Read the model definition and answer for the solid it produces. Units are mm, in the model's axes. A direction names the side the tool comes from. Give positions to 0.01 mm unless a question says otherwise; leave off trailing zeros. Loops run counter-clockwise (first coordinate to the right, second up) from the corner with the lowest first, then second, coordinate; pieces in that order, holes last. Notation, with made-up numbers: (3.5, 14) - (42.5, 14) arc R17 ccw to (42.5, 20) - close; hole circle Ø7 at (-37, 10.25). An arc over 180 degrees is marked (long way). Use a Markdown table: item, result. Add a question column.
Item 1: A cutting plane is placed at A-A (y = 124.5). Determine the outline of the cut face in (x, z).
Item 2: Which of the six approach directions +Z, -Z, +X, -X, +Y, -Y give full straight-line access (tool end or side, diameter ignored) to faces 1 (the face through (128.614, 56.311, 3.944)), 2 (the face through (37.56, 139.12, 4.54)), 3 (the face through (70, 0, 4))?
Item 3: For a pull along Z with two mould halves and no side action, classify faces 4 (the face through (71, 73, 8)), 5 (the face through (137, 134.052, 4)), 6 (the face through (140.936, 27.363, 3.944)) as +Z half, -Z half, draft (parallel to the pull), parting line (faces both ways), or undercut.
Item 4: A cutting plane is placed at B-B (x = 70). Determine the outline of the cut face in (y, z).
Item 5: A cutting plane is placed at C-C (y = 56.5). Determine the outline of the cut face in (x, z), plus the area to 3 significant figures.
Item 6: Consider probe 1 along X at (y, z) = (78, 0.75); probe 2 along Y at (x, z) = (117, 2); probe 3 along Y at (x, z) = (100.5, 1.75). Determine where each line is inside the solid, lowest interval first. Write a range as [from, to].
Item 7: A cutting plane is placed at D-D (x = 40). Determine the outline of the cut face in (y, z).
Item 8: Each of these flat-tipped pins is pushed along its axis until it touches: P1, Ø2, axis at x = 46.5, z = 2, coming from the -Y side; P2, Ø1.5, axis at x = 101, z = 3.5, coming from the +Y side; P3, Ø0.9, axis at x = 123.5, z = 5.5, coming from the +Y side. Where does it stop, or does it pass through?
from build123d import *

# Parameters (mm, degrees)
BOSS_EXTRUDE1_DEPTH    = 8
SPLIT1_SURFACE_1_BACK  = 343.199
SPLIT1_SURFACE_1_DEPTH = 686.398
SPLIT1_SURFACE_2_BACK  = 343.199
SPLIT1_SURFACE_2_DEPTH = 686.398
SKETCH5_R              = 2.5
CUT_EXTRUDE6_DEPTH     = 10
SKETCH4_R              = 2.5
CUT_EXTRUDE7_DEPTH     = 10
SKETCH6_R              = 1.5
CUT_EXTRUDE8_DEPTH     = 342.206659287
SKETCH7_W              = 49
SKETCH7_H              = 49
SKETCH7_W_2            = 18
SKETCH7_H_2            = 18
BOSS_EXTRUDE2_DEPTH    = 15
SKETCH8_W              = 49
SKETCH8_H              = 49
SKETCH8_R              = 1.5
BOSS_EXTRUDE3_DEPTH    = 10
SKETCH9_W              = 49
SKETCH9_H              = 49
CUT_EXTRUDE9_DEPTH     = 8
SKETCH10_W             = 49
SKETCH10_H             = 49
SKETCH10_W_2           = 18
SKETCH10_H_2           = 18
BOSS_EXTRUDE4_DEPTH    = 8
SKETCH12_R             = 2.5
CUT_EXTRUDE10_DEPTH    = 343.027753759


with BuildPart() as part:
    # Sketch1 → Boss-Extrude1 (new body)
    with BuildSketch(Plane.XY):
        with BuildLine():
            Line((70, 309.985818768), (85.299227191, 309.985818768))
            ThreePointArc((85.299227191, 309.985818768), (88.489017574, 308.836174247), (90.211957942, 305.915913694))
            Line((90.211957942, 305.915913694), (96.672728921, 271.790334282))
            ThreePointArc((96.672728921, 271.790334282), (97.06575438, 270.906904614), (97.621470019, 270.115641625))
            Line((97.621470019, 270.115641625), (139.950460317, 220.786053348))
            ThreePointArc((139.950460317, 220.786053348), (141.739336996, 217.746026552), (142.361429131, 214.274017901))
            Line((142.361429131, 214.274017901), (142.361429131, 30.859943174))
            ThreePointArc((142.361429131, 30.859943174), (140.896963037, 27.324409268), (137.361429131, 25.859943174))
            Line((137.361429131, 25.859943174), (114.717190871, 25.782318449))
            ThreePointArc((114.717190871, 25.782318449), (112.681998989, 25.341726514), (111.002773989, 24.110332733))
            Line((111.002773989, 24.110332733), (89.38285929, 0))
            Line((89.38285929, 0), (50.5, 0))
            Line((50.5, 0), (28.997226011, 24.110332733))
            ThreePointArc((28.997226011, 24.110332733), (27.318001011, 25.341726514), (25.282809129, 25.782318449))
            Line((25.282809129, 25.782318449), (2.638570869, 25.859943174))
            ThreePointArc((2.638570869, 25.859943174), (-0.896963037, 27.324409268), (-2.361429131, 30.859943174))
            Line((-2.361429131, 30.859943174), (-2.361429131, 214.274017901))
            ThreePointArc((-2.361429131, 214.274017901), (-1.739336996, 217.746026552), (0.049539683, 220.786053348))
            Line((0.049539683, 220.786053348), (42.261389271, 270.115641625))
            ThreePointArc((42.261389271, 270.115641625), (42.81710491, 270.906904614), (43.210130369, 271.790334282))
            Line((43.210130369, 271.790334282), (49.724618218, 305.923183314))
            ThreePointArc((49.724618218, 305.923183314), (51.449026762, 308.838533573), (54.635967087, 309.985818768))
            Line((54.635967087, 309.985818768), (70, 309.985818768))
        make_face()
        with BuildLine():
            Line((15.218798766, 54.807228462), (17.702103505, 54.807228462))
            ThreePointArc((17.702103505, 54.807228462), (21.420312934, 56.347361236), (22.960445707, 60.065570665))
            Line((22.960445707, 60.065570665), (22.960445707, 189.807228462))
            ThreePointArc((22.960445707, 189.807228462), (21.495979613, 193.342762368), (17.960445707, 194.807228462))
            Line((17.960445707, 194.807228462), (14.960456564, 194.807228462))
            ThreePointArc((14.960456564, 194.807228462), (11.424922658, 193.342762368), (9.960456564, 189.807228462))
            Line((9.960456564, 189.807228462), (9.960456564, 60.065570665))
            ThreePointArc((9.960456564, 60.065570665), (11.500589337, 56.347361236), (15.218798766, 54.807228462))
        make_face(mode=Mode.SUBTRACT)
        with BuildLine():
            Line((125.039543436, 54.807228462), (122.039554293, 54.807228462))
            ThreePointArc((122.039554293, 54.807228462), (118.504020387, 56.271694556), (117.039554293, 59.807228462))
            Line((117.039554293, 59.807228462), (117.039554293, 189.807228462))
            ThreePointArc((117.039554293, 189.807228462), (118.504020387, 193.342762368), (122.039554293, 194.807228462))
            Line((122.039554293, 194.807228462), (125.039543436, 194.807228462))
            ThreePointArc((125.039543436, 194.807228462), (128.575077342, 193.342762368), (130.039543436, 189.807228462))
            Line((130.039543436, 189.807228462), (130.039543436, 59.807228462))
            ThreePointArc((130.039543436, 59.807228462), (128.575077342, 56.271694556), (125.039543436, 54.807228462))
        make_face(mode=Mode.SUBTRACT)
    extrude(amount=BOSS_EXTRUDE1_DEPTH)


with BuildPart() as body_2:
    # Split1: the piece behind the surface
    add(part.part)
    # Split1 surface: a surface, the sketch's curves swept straight by 686.398 mm
    with BuildLine(Plane(origin=(0, 0, 0), x_dir=(-1, 0, 0), z_dir=(0, 0, -1)).offset(-SPLIT1_SURFACE_1_BACK), mode=Mode.PRIVATE) as split1_surface_1_path:
        Line((-142.361429131, 144.05225917), (2.361429131, 144.05225917))
    split1_surface_1 = Shell.extrude(split1_surface_1_path.wire(), (0 * SPLIT1_SURFACE_1_DEPTH, 0 * SPLIT1_SURFACE_1_DEPTH, -1 * SPLIT1_SURFACE_1_DEPTH))
    split(bisect_by=split1_surface_1, keep=Keep.BOTTOM)

    # Sketch5 → Cut-Extrude6 (cut)
    with BuildSketch(Plane(origin=(0, 144.05225917, -115.359943174), x_dir=(1, 0, 0), z_dir=(0, -1, 0))):
        with Locations(Location((70, 119.359943174, 0), (0, 0, 270))):
            Circle(SKETCH5_R)
        with Locations(Location((100, 119.359943174, 0), (0, 0, 270))):
            Circle(SKETCH5_R)
        with Locations(Location((40, 119.359943174, 0), (0, 0, 270))):
            Circle(SKETCH5_R)
        with Locations(Location((2.638570869, 119.359943174, 0), (0, 0, 270))):
            Circle(SKETCH5_R)
        with Locations(Location((137.361429131, 119.359943174, 0), (0, 0, 270))):
            Circle(SKETCH5_R)
    extrude(amount=CUT_EXTRUDE6_DEPTH, mode=Mode.SUBTRACT)


with BuildPart() as part_1:
    add(part.part)

    # Split1: split by a surface, the side it looks to stays
    # Split1 surface: a surface, the sketch's curves swept straight by 686.398 mm
    with BuildLine(Plane(origin=(0, 0, 0), x_dir=(-1, 0, 0), z_dir=(0, 0, -1)).offset(-SPLIT1_SURFACE_2_BACK), mode=Mode.PRIVATE) as split1_surface_2_path:
        Line((-142.361429131, 144.05225917), (2.361429131, 144.05225917))
    split1_surface_2 = Shell.extrude(split1_surface_2_path.wire(), (0 * SPLIT1_SURFACE_2_DEPTH, 0 * SPLIT1_SURFACE_2_DEPTH, -1 * SPLIT1_SURFACE_2_DEPTH))
    split(bisect_by=split1_surface_2, keep=Keep.TOP)

    # Sketch4 → Cut-Extrude7 (cut)
    with BuildSketch(Plane(origin=(0, 144.05225917, 0), x_dir=(-1, 0, 0), z_dir=(0, -1, 0))):
        with Locations(Location((-70, -4, 0), (0, 0, 90))):
            Circle(SKETCH4_R)
        with Locations(Location((-40, -4, 0), (0, 0, 90))):
            Circle(SKETCH4_R)
        with Locations(Location((-100, -4, 0), (0, 0, 90))):
            Circle(SKETCH4_R)
        with Locations(Location((-137.361429131, -4, 0), (0, 0, 90))):
            Circle(SKETCH4_R)
        with Locations(Location((-3.799513716, -4, 0), (0, 0, 270))):
            Circle(SKETCH4_R)
    extrude(amount=-CUT_EXTRUDE7_DEPTH, mode=Mode.SUBTRACT)

    # Sketch6 → Cut-Extrude8 (cut, through all)
    with BuildSketch(Plane.XY.offset(8)):
        with Locations((50.000130369, 267.980334282)):
            Circle(SKETCH6_R)
        with Locations((90.000130369, 267.980334282)):
            Circle(SKETCH6_R)
        with Locations((90.000130369, 227.980334282)):
            Circle(SKETCH6_R)
        with Locations((50.000130369, 227.980334282)):
            Circle(SKETCH6_R)
    extrude(amount=-CUT_EXTRUDE8_DEPTH, mode=Mode.SUBTRACT)

    # Sketch7 → Boss-Extrude2 (add)
    with BuildSketch(Plane(origin=(0, 0, 0), x_dir=(-1, 0, 0), z_dir=(0, 0, -1))):
        with Locations((-70.000130369, 247.980334282)):
            Rectangle(SKETCH7_W, SKETCH7_H)
        with Locations((-56.000130369, 261.980334282)):
            Rectangle(SKETCH7_W_2, SKETCH7_H_2, mode=Mode.SUBTRACT)
        with Locations((-84.000130369, 261.980334282)):
            Rectangle(SKETCH7_W_2, SKETCH7_H_2, mode=Mode.SUBTRACT)
        with Locations((-84.000130369, 233.980334282)):
            Rectangle(SKETCH7_W_2, SKETCH7_H_2, mode=Mode.SUBTRACT)
        with Locations((-56.000130369, 233.980334282)):
            Rectangle(SKETCH7_W_2, SKETCH7_H_2, mode=Mode.SUBTRACT)
    extrude(amount=BOSS_EXTRUDE2_DEPTH)

    # Sketch8 → Boss-Extrude3 (add)
    with BuildSketch(Plane(origin=(0, 0, -15), x_dir=(-1, 0, 0), z_dir=(0, 0, -1))):
        with Locations((-70.000130369, 247.980334282)):
            Rectangle(SKETCH8_W, SKETCH8_H)
        with Locations(Location((-50.000130369, 267.980334282, 0), (0, 0, 180))):
            Circle(SKETCH8_R, mode=Mode.SUBTRACT)
        with Locations(Location((-90.000130369, 267.980334282, 0), (0, 0, 180))):
            Circle(SKETCH8_R, mode=Mode.SUBTRACT)
        with Locations(Location((-50.000130369, 227.980334282, 0), (0, 0, 180))):
            Circle(SKETCH8_R, mode=Mode.SUBTRACT)
        with Locations(Location((-90.000130369, 227.980334282, 0), (0, 0, 180))):
            Circle(SKETCH8_R, mode=Mode.SUBTRACT)
    extrude(amount=BOSS_EXTRUDE3_DEPTH)

    # Sketch9 → Cut-Extrude9 (cut)
    with BuildSketch(Plane.XY.offset(8)):
        with Locations((70.000130369, 247.980334282)):
            Rectangle(SKETCH9_W, SKETCH9_H)
    extrude(amount=-CUT_EXTRUDE9_DEPTH, mode=Mode.SUBTRACT)


with BuildPart() as cut_extrude9_piece_1:
    # of the separate pieces the step leaves, piece 1, a body of its own (cut_extrude9_pieces)
    add(part_1.part.solids().sort_by_distance((49.724618218, 305.923183314, 0))[0])



with BuildPart() as cut_extrude9_piece_2:
    # of the separate pieces the step leaves, piece 2, a body of its own (cut_extrude9_pieces)
    add(part_1.part.solids().sort_by_distance((45.500130369, 223.480334282, -25))[0])


with BuildPart() as cut_extrude9_piece_1_1:
    add(cut_extrude9_piece_1.part)

    add(cut_extrude9_piece_2.part)  # Boss-Extrude4 merges Cut-Extrude9 piece 2
    # Sketch10 → Boss-Extrude4 (add)
    with BuildSketch(Plane.XY):
        with Locations((70.000130369, 247.980334282)):
            Rectangle(SKETCH10_W, SKETCH10_H)
        with Locations((84.000130369, 261.980334282)):
            Rectangle(SKETCH10_W_2, SKETCH10_H_2, mode=Mode.SUBTRACT)
        with Locations((56.000130369, 261.980334282)):
            Rectangle(SKETCH10_W_2, SKETCH10_H_2, mode=Mode.SUBTRACT)
        with Locations((56.000130369, 233.980334282)):
            Rectangle(SKETCH10_W_2, SKETCH10_H_2, mode=Mode.SUBTRACT)
        with Locations((84.000130369, 233.980334282)):
            Rectangle(SKETCH10_W_2, SKETCH10_H_2, mode=Mode.SUBTRACT)
    extrude(amount=BOSS_EXTRUDE4_DEPTH)

    # Sketch12 → Cut-Extrude10 (cut, through all)
    with BuildSketch(Plane(origin=(0, 0, 0), x_dir=(-1, 0, 0), z_dir=(0, 0, -1))):
        with Locations((-102.960445707, 197.503395095)):
            Circle(SKETCH12_R)
        with Locations((-35.960445707, 197.503395095)):
            Circle(SKETCH12_R)
        with Locations((-35.960445707, 157.503395095)):
            Circle(SKETCH12_R)
        with Locations((-102.960445707, 157.503395095)):
            Circle(SKETCH12_R)
    extrude(amount=-CUT_EXTRUDE10_DEPTH, mode=Mode.SUBTRACT)


solid = body_2.part
Geometry says:
| question | item | result |
|---|---|---|
| 1 | outline | (-2.36, 0) - (9.96, 0) - (9.96, 8) - (-2.36, 8) - close; (22.96, 0) - (117.04, 0) - (117.04, 8) - (22.96, 8) - close; (130.04, 0) - (142.36, 0) - (142.36, 8) - (130.04, 8) - close |
| 2 | face 1 | +Z, -Z, +Y |
| 2 | face 2 | +Y |
| 2 | face 3 | +Z, -Z, +X, -X, -Y |
| 3 | face 4 | +Z half |
| 3 | face 5 | undercut |
| 3 | face 6 | draft |
| 4 | outline | (0, 0) - (144.05, 0) - (144.05, 1.5) - (134.05, 1.5) - (134.05, 6.5) - (144.05, 6.5) - (144.05, 8) - (0, 8) - close |
| 5 | outline | (-2.36, 0) - (11.35, 0) - (11.35, 8) - (-2.36, 8) - close; (21.57, 0) - (118.29, 0) - (118.29, 8) - (21.57, 8) - close; (128.79, 0) - (142.36, 0) - (142.36, 8) - (128.79, 8) - close |
| 5 | area | 992 mm² |
| 6 | probe 1 | [-2.36, 9.96], [22.96, 117.04], [130.04, 142.36] |
| 6 | probe 2 | [25.79, 144.05] |
| 6 | probe 3 | [12.4, 134.05] |
| 7 | outline | (11.77, 0) - (144.05, 0) - (144.05, 1.5) - (134.05, 1.5) - (134.05, 6.5) - (144.05, 6.5) - (144.05, 8) - (11.77, 8) - close |
| 8 | P1 | y = 3.36 |
| 8 | P2 | y = 134.05 |
| 8 | P3 | y = 54.81 |
